```python
from build123d import *

# Parameters (mm, degrees)
BOSS_EXTRUDE1_DEPTH = 140
SKETCH2_R           = 4
CUT_EXTRUDE1_DEPTH  = 10


with BuildPart() as part:
    # Sketch1 → Boss-Extrude1 (new body)
    with BuildSketch(Plane.YZ):
        Polygon((60, 0), (-60, 0), (-127, -67), (-130, -67), (-60, 3), (60, 3), (130, -67), (127, -67), align=None)
    extrude(amount=BOSS_EXTRUDE1_DEPTH)

    # Sketch2 → Cut-Extrude1 (cut)
    with BuildSketch(Plane(origin=(0, 0, 0), x_dir=(1, 0, 0), z_dir=(0, 0, -1))):
        with Locations(Location((30, 0, 0), (0, 0, 270))):
            Circle(SKETCH2_R)
        with Locations(Location((110, 0, 0), (0, 0, 270))):
            Circle(SKETCH2_R)
        with Locations(Location((70, 30, 0), (0, 0, 270))):
            Circle(SKETCH2_R)
        with Locations(Location((70, -30, 0), (0, 0, 270))):
            Circle(SKETCH2_R)
    extrude(amount=-CUT_EXTRUDE1_DEPTH, mode=Mode.SUBTRACT)


solid = part.part
```
For this review, take the finished solid that the model builds, in its own axes (mm). A direction names the side the tool comes from. Round coordinates to 2 decimals unless told otherwise and drop trailing zeros. Write each loop counter-clockwise with the first axis right and the second up, starting at its lowest first coordinate (ties: lowest second). Pieces come first, ordered by that corner, then holes.
1) Take a section at D-D on y = -79. Give the boundary of the cut face in (x, z).
Answer below:
outline: (0, -19) - (140, -19) - (140, -16) - (0, -16) - close
2) Machinability: for faces 5 (the face through (69, -95, -32)), 6 (the face through (69, 94, -34)), which of the approach directions +Z, -Z, +X, -X, +Y, -Y give a long, thin tool a straight path to every point of the face, cutting with its end or side? Answer none if there is none.
Answer below:
face 5: +Z, +X, -X, -Y
face 6: -Z, +X, -X
3) Take a section at B-B on z = -53. Give the boundary of the cut face in (x, y).
Answer below:
outline: (0, -116) - (140, -116) - (140, -113) - (0, -113) - close; (0, 113) - (140, 113) - (140, 116) - (0, 116) - close
4) Mouldability with a two-part tool opening along X and no side actions: class faces 1 (the face through (69, -93, -33)), 2 (the face through (66.095, -30.867, 1.479)), 3 (the face through (140, 1, 2)), 4 (the face through (33.966, -0.521, 1.479)) as +X half, -X half, draft (parallel to the pull), parting line (faces both ways), or undercut.
Answer below:
face 1: draft
face 2: undercut
face 3: +X half
face 4: undercut
5) Take a section at C-C on y = 30. Give the boundary of the cut face in (x, z).
Answer below:
outline: (0, 0) - (66, 0) - (66, 3) - (0, 3) - close; (74, 0) - (140, 0) - (140, 3) - (74, 3) - close
6) Take a section at A-A on x = 110. Give the boundary of the cut face in (y, z).
Answer below:
outline: (-130, -67) - (-127, -67) - (-60, 0) - (-4, 0) - (-4, 3) - (-60, 3) - close; (4, 0) - (60, 0) - (127, -67) - (130, -67) - (60, 3) - (4, 3) - close
7) For line 1 along X through (y, z) = (0, 1.5); line 2 along X through (y, z) = (30, 0.85); line 3 along Z through (x, y) = (125.5, -19), list the stretches that pass through material, from the lowest coordinate up.
Answer below:
line 1: x = 0 to 26, 34 to 106, 114 to 140
line 2: x = 0 to 66, 74 to 140
line 3: z = 0 to 3
8) Insertion check: pin 1 Ø13 at (x, y) = (110, 0) entering from -Z; pin 2 Ø3 at (x, z) = (18.5, -40) entering from +Y; pin 3 Ø12 at (x, z) = (55, -41.5) entering from +Y; pin 4 Ø7 at (x, y) = (70, -30) entering from -Z. Each pin has a flat end and moves straight along its axis. Give the tip position at first contact, or say it passes through.
Answer below:
pin 1: stops at z = 0
pin 2: stops at y = 104.5
pin 3: stops at y = 110.5
pin 4: passes through
